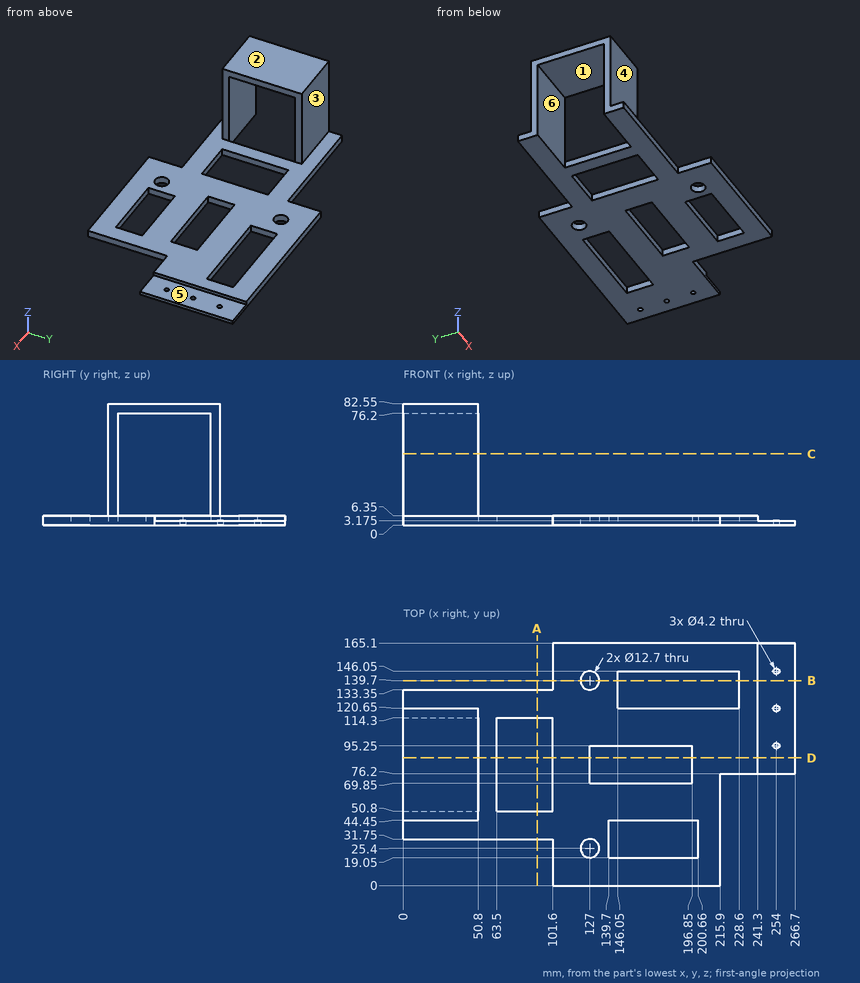
Answer from the drawing. Dimensions are ordinates in mm from the lowest x, y and z of the part. A direction names the side the tool comes from. Round coordinates to 2 decimals unless told otherwise and drop trailing zeros. Write each loop counter-clockwise with the first axis right and the second up, starting at its lowest first coordinate (ties: lowest second). Pieces come first, ordered by that corner, then holes. Notation, with made-up numbers: M -22.5,-25.5 L -3.5,-25.5 A14 ccw -3.5,-16.5 Z; hole C 40.25,37 d2. An arc over 180 degrees is marked long. Write each question's results on one line, items separated by ' | '. Start each with the question number.
Item 1: Which of the six approach directions +Z, -Z, +X, -X, +Y, -Y give full straight-line access (tool end or side, diameter ignored) to the marked faces 1, 2 and 3?
Item 2: Find section D-D on y = 87. Write down the section's boundary in (x, z) (3 decimals), and give its area (3 significant figures).
Item 3: The mould has two halves that part along Y. Classify the marked faces 4, 5 and 6: +Y half, -Y half, draft (parallel to the pull), parting line (faces both ways), or undercut.
Item 4: Find section C-C on z = 48.5. Write down the section's boundary in (x, y), and give its area (3 significant figures).
Item 5: Find section A-A on x = 91. Write down the section's boundary in (y, z).
Item 6: Straight lines are drawn through the part: probe 1 along Y at (x, z) = (254, 1); probe 2 along X at (y, z) = (139, 3); probe 3 along Y at (x, z) = (42, 54.5). For each, find the intervals that lie inside material, in ascending order.
Item 7: Find section B-B on y = 139.7. Write down the section's boundary in (x, z) (3 decimals), and give its area (3 significant figures).
Item 8: Given pin 1 Ø7 at (x, z) = (42, 4.5) entering from -Y; pin 2 Ø7 at (y, z) = (80.5, 3.5) entering from -X; pin 3 Ø5 at (x, y) = (45.5, 95.5) entering from -Z, each flat-ended and moving along its own axis, determine where each tip first touches the part or whether it passes through.
Answer block:
1) face 1: -Z, +X, -X | face 2: +Z, +X, -X, +Y, -Y | face 3: +Z, +X, -X, +Y
2) outline: M 0,76.2 L 50.8,76.2 L 50.8,82.55 L 0,82.55 Z; M 50.8,0 L 63.5,0 L 63.5,6.35 L 50.8,6.35 Z; M 101.6,0 L 127,0 L 127,6.35 L 101.6,6.35 Z; M 196.85,0 L 266.7,0 L 266.7,3.175 L 241.3,3.175 L 241.3,6.35 L 196.85,6.35 Z | area: 927 mm²
3) face 4: -Y half | face 5: draft | face 6: undercut
4) outline: M 0,44.45 L 50.8,44.45 L 50.8,50.8 L 0,50.8 Z; M 0,114.3 L 50.8,114.3 L 50.8,120.65 L 0,120.65 Z | area: 645 mm²
5) outline: M 31.75,0 L 50.8,0 L 50.8,6.35 L 31.75,6.35 Z; M 114.3,0 L 133.35,0 L 133.35,6.35 L 114.3,6.35 Z
6) probe 1: y = 76.2 to 93.15, 97.35 to 118.55, 122.75 to 143.95, 148.15 to 165.1 | probe 2: x = 101.6 to 120.69, 133.31 to 146.05, 228.6 to 266.7 | probe 3: y = 44.45 to 50.8, 114.3 to 120.65
7) outline: M 101.6,0 L 120.65,0 L 120.65,6.35 L 101.6,6.35 Z; M 133.35,0 L 146.05,0 L 146.05,6.35 L 133.35,6.35 Z; M 228.6,0 L 266.7,0 L 266.7,3.175 L 241.3,3.175 L 241.3,6.35 L 228.6,6.35 Z | area: 363 mm²
8) pin 1: stops at y = 31.75 | pin 2: stops at x = 50.8 | pin 3: stops at z = 76.2
